Check sheet for the modelled part. Datum: model origin and axes. Units: mm. Face numbers are marked on the shaded views. A direction names the side the tool comes from. Give positions to 0.01 mm unless a question says otherwise; leave off trailing zeros. Order: outer loops, then holes, each group sorted by start corner. A loop starts at its lowest first (then second) coordinate and runs counter-clockwise, first axis right, second up.
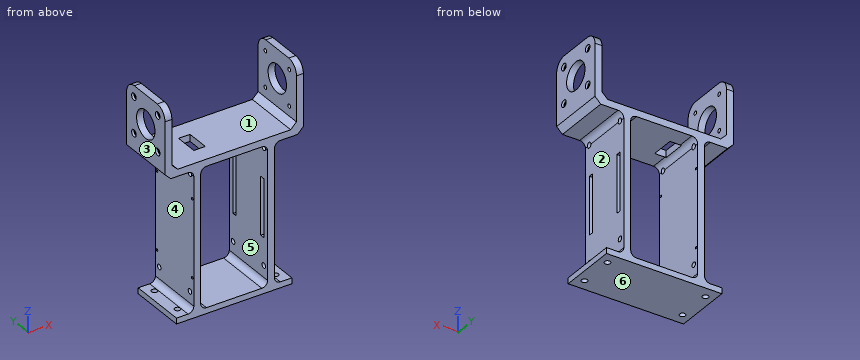
```python
from build123d import *

# Parameters (mm, degrees)
SKETCH1_W           = 120
SKETCH1_H           = 65
SKETCH1_W_2         = 108
SKETCH1_H_2         = 54
BOSS_EXTRUDE1_DEPTH = 50
SKETCH4_R           = 12
CUT_EXTRUDE1_DEPTH  = 156
SKETCH7_R           = 1.735318072
CUT_EXTRUDE2_DEPTH  = 156
SKETCH9_R           = 3
CUT_EXTRUDE3_DEPTH  = 2
CUT_EXTRUDE4_START  = -2
SKETCH10_R          = 3
CUT_EXTRUDE4_DEPTH  = 2
SKETCH11_W          = 6
SKETCH11_H          = 50
BOSS_EXTRUDE2_DEPTH = 120
SKETCH13_W          = 120
SKETCH13_H          = 5
CUT_EXTRUDE5_DEPTH  = 120
FILLET1_R           = 10
SKETCH14_W          = 100
SKETCH14_H          = 50
BOSS_EXTRUDE3_DEPTH = 5
SKETCH15_R          = 2.5
CUT_EXTRUDE6_DEPTH  = 18
SKETCH16_W          = 50
SKETCH16_H          = 4
CUT_EXTRUDE7_DEPTH  = 18
SKETCH17_R          = 1
CUT_EXTRUDE8_DEPTH  = 18
SKETCH18_W          = 10
SKETCH18_H          = 20
CUT_EXTRUDE9_DEPTH  = 18
SKETCH22_R          = 2.25
CUT_EXTRUDE13_DEPTH = 75
CHAMFER1_SIZE       = 5
CHAMFER2_SIZE       = 5
FILLET2_R           = 5


with BuildPart() as part:
    # Sketch1 → Boss-Extrude1 (new body)
    with BuildSketch(Plane(origin=(0, 0, 0), x_dir=(1, 0, 0), z_dir=(0, 1, 0))):
        with Locations((0, 2.5)):
            Rectangle(SKETCH1_W, SKETCH1_H)
        with Locations((0, 2)):
            Rectangle(SKETCH1_W_2, SKETCH1_H_2, mode=Mode.SUBTRACT)
    extrude(amount=BOSS_EXTRUDE1_DEPTH)

    # Sketch4 → Cut-Extrude1 (cut)
    with BuildSketch(Plane.ZY.offset(60)):
        with Locations((0, 25)):
            Circle(SKETCH4_R)
    extrude(amount=-CUT_EXTRUDE1_DEPTH, mode=Mode.SUBTRACT)

    # Sketch7 → Cut-Extrude2 (cut)
    with BuildSketch(Plane.ZY.offset(60)):
        with Locations((-15.5, 9.5)):
            Circle(SKETCH7_R)
        with Locations((-15.5, 40.5)):
            Circle(SKETCH7_R)
        with Locations((15.5, 9.5)):
            Circle(SKETCH7_R)
        with Locations((15.5, 40.5)):
            Circle(SKETCH7_R)
    extrude(amount=-CUT_EXTRUDE2_DEPTH, mode=Mode.SUBTRACT)

    # Sketch9 → Cut-Extrude3 (cut)
    with BuildSketch(Plane(origin=(60, 0, 0), x_dir=(0, 0, -1), z_dir=(1, 0, 0))):
        with Locations((15.5, 40.5)):
            Circle(SKETCH9_R)
        with Locations((15.5, 9.5)):
            Circle(SKETCH9_R)
        with Locations((-15.5, 9.5)):
            Circle(SKETCH9_R)
        with Locations((-15.5, 40.5)):
            Circle(SKETCH9_R)
    extrude(amount=-CUT_EXTRUDE3_DEPTH, mode=Mode.SUBTRACT)

    # Sketch10 → Cut-Extrude4 (cut)
    with BuildSketch(Plane.ZY.offset(60).offset(CUT_EXTRUDE4_START)):
        with Locations(Location((-15.5, 9.5, 0), (0, 0, 180))):
            Circle(SKETCH10_R)
        with Locations(Location((-15.5, 40.5, 0), (0, 0, 180))):
            Circle(SKETCH10_R)
        with Locations(Location((15.5, 40.5, 0), (0, 0, 180))):
            Circle(SKETCH10_R)
        with Locations(Location((15.5, 9.5, 0), (0, 0, 180))):
            Circle(SKETCH10_R)
    extrude(amount=CUT_EXTRUDE4_DEPTH, mode=Mode.SUBTRACT)

    # Sketch11 → Boss-Extrude2 (add)
    with BuildSketch(Plane(origin=(0, 0, -35), x_dir=(-1, 0, 0), z_dir=(0, 0, -1))):
        with Locations((-32, 25)):
            Rectangle(SKETCH11_W, SKETCH11_H)
        with Locations((32, 25)):
            Rectangle(SKETCH11_W, SKETCH11_H)
    extrude(amount=BOSS_EXTRUDE2_DEPTH)

    # Sketch13 → Cut-Extrude5 (cut)
    with BuildSketch(Plane(origin=(0, 50, 0), x_dir=(1, 0, 0), z_dir=(0, 1, 0))):
        with Locations((0, -27.5)):
            Rectangle(SKETCH13_W, SKETCH13_H)
    extrude(amount=-CUT_EXTRUDE5_DEPTH, mode=Mode.SUBTRACT)

    # Fillet1
    fillet1_edges = [part.edges().sort_by_distance(p)[0] for p in [
        (57, 0, 25),
        (-57, 0, 25),
        (57, 50, 25),
        (-57, 50, 25),
    ]]
    fillet(fillet1_edges, radius=FILLET1_R)

    # Sketch14 → Boss-Extrude3 (add)
    with BuildSketch(Plane(origin=(0, 0, -155), x_dir=(-1, 0, 0), z_dir=(0, 0, -1))):
        with Locations((0, 25)):
            Rectangle(SKETCH14_W, SKETCH14_H)
    extrude(amount=BOSS_EXTRUDE3_DEPTH)

    # Sketch15 → Cut-Extrude6 (cut)
    with BuildSketch(Plane(origin=(0, 0, -160), x_dir=(-1, 0, 0), z_dir=(0, 0, -1))):
        with Locations((-42.5, 10)):
            Circle(SKETCH15_R)
        with Locations((42.5, 10)):
            Circle(SKETCH15_R)
        with Locations((42.5, 40)):
            Circle(SKETCH15_R)
        with Locations((-42.5, 40)):
            Circle(SKETCH15_R)
    extrude(amount=-CUT_EXTRUDE6_DEPTH, mode=Mode.SUBTRACT)

    # Sketch16 → Cut-Extrude7 (cut)
    with BuildSketch(Plane(origin=(35, 0, 0), x_dir=(0, 0, -1), z_dir=(1, 0, 0))):
        with Locations((91.261804775, 43)):
            Rectangle(SKETCH16_W, SKETCH16_H)
        with Locations((91.261804775, 7)):
            Rectangle(SKETCH16_W, SKETCH16_H)
    extrude(amount=-CUT_EXTRUDE7_DEPTH, mode=Mode.SUBTRACT)

    # Sketch17 → Cut-Extrude8 (cut)
    with BuildSketch(Plane.ZY.offset(35)):
        with Locations(Location((-127, 2, 0), (0, 0, 270))):
            Circle(SKETCH17_R)
        with Locations(Location((-127, 48, 0), (0, 0, 270))):
            Circle(SKETCH17_R)
        with Locations(Location((-60, 2, 0), (0, 0, 270))):
            Circle(SKETCH17_R)
        with Locations(Location((-60, 48, 0), (0, 0, 270))):
            Circle(SKETCH17_R)
    extrude(amount=-CUT_EXTRUDE8_DEPTH, mode=Mode.SUBTRACT)

    # Sketch18 → Cut-Extrude9 (cut)
    with BuildSketch(Plane(origin=(0, 0, -35), x_dir=(-1, 0, 0), z_dir=(0, 0, -1))):
        with Locations((20, 25)):
            Rectangle(SKETCH18_W, SKETCH18_H)
    extrude(amount=-CUT_EXTRUDE9_DEPTH, mode=Mode.SUBTRACT)

    # Sketch22 → Cut-Extrude13 (cut)
    with BuildSketch(Plane.ZY.offset(35)):
        with Locations(Location((-140, 5, 0), (0, 0, 270))):
            Circle(SKETCH22_R)
        with Locations(Location((-140, 45, 0), (0, 0, 270))):
            Circle(SKETCH22_R)
        with Locations(Location((-40, 5, 0), (0, 0, 270))):
            Circle(SKETCH22_R)
        with Locations(Location((-40, 45, 0), (0, 0, 270))):
            Circle(SKETCH22_R)
    extrude(amount=-CUT_EXTRUDE13_DEPTH, mode=Mode.SUBTRACT)

    # Chamfer1
    chamfer1_edges = [part.edges().sort_by_distance(p)[0] for p in [
        (-60, 25, -35),
        (60, 25, -35),
    ]]
    chamfer(chamfer1_edges, length=CHAMFER1_SIZE)

    # Chamfer2
    chamfer2_edges = [part.edges().sort_by_distance(p)[0] for p in [
        (-54, 25, -29),
        (54, 25, -29),
    ]]
    chamfer(chamfer2_edges, length=CHAMFER2_SIZE)

    # Fillet2
    # the kernel refuses this fillet: 5 mm, written as the material it adds along each edge
    with BuildSketch(Plane(origin=(-29, 50, -155), x_dir=(1, 0, 0), z_dir=(0, -1, 0)), Plane(origin=(29, 0, -155), x_dir=(-1, 0, 0), z_dir=(0, 1, 0))) as fillet2_piece_1:
        with BuildLine():
            CenterArc((FILLET2_R, FILLET2_R), FILLET2_R, 180, 90)
            Line((0, FILLET2_R), (0, 0))
            Line((0, 0), (FILLET2_R, 0))
        make_face()
    extrude(amount=50)
    with BuildSketch(Plane(origin=(35, 50, -35), x_dir=(1, 0, 0), z_dir=(0, -1, 0))) as fillet2_piece_2_section:
        with BuildLine():
            CenterArc((FILLET2_R, -FILLET2_R), FILLET2_R, 90, 90)
            Line((0, -FILLET2_R), (0, 0))
            Line((0, 0), (FILLET2_R, 0))
        make_face()
    fillet2_piece_2 = extrude(amount=50, mode=Mode.PRIVATE)
    fillet2_piece_2 = fillet2_piece_2 - Plane(origin=(36.144503009, 45, -40), x_dir=(0, -1, 0), z_dir=(-1, 0, 0)) * Cylinder(2.25, 121, mode=Mode.PRIVATE)
    fillet2_piece_2 = fillet2_piece_2 - Plane(origin=(36.144503009, 5, -40), x_dir=(0, -1, 0), z_dir=(-1, 0, 0)) * Cylinder(2.25, 121, mode=Mode.PRIVATE)
    add(fillet2_piece_2)
    with BuildSketch(Plane(origin=(-29, 50, -35), x_dir=(0, 0, -1), z_dir=(0, -1, 0))) as fillet2_piece_3_section:
        with BuildLine():
            CenterArc((FILLET2_R, FILLET2_R), FILLET2_R, 180, 90)
            Line((0, FILLET2_R), (0, 0))
            Line((0, 0), (FILLET2_R, 0))
        make_face()
    fillet2_piece_3 = extrude(amount=50, mode=Mode.PRIVATE)
    fillet2_piece_3 = fillet2_piece_3 - Plane(origin=(-27.918643219, 45, -40), x_dir=(0, -1, 0), z_dir=(-1, 0, 0)) * Cylinder(2.25, 121, mode=Mode.PRIVATE)
    fillet2_piece_3 = split(fillet2_piece_3, bisect_by=Plane(origin=(-27.918643219, 35, -36.105806531), z_dir=(0, 1, 0)), keep=Keep.TOP, mode=Mode.PRIVATE)
    fillet2_piece_3 = split(fillet2_piece_3, bisect_by=Plane(origin=(-25, 42.450189762, -36.105806531), z_dir=(-1, 0, 0)), keep=Keep.TOP, mode=Mode.PRIVATE)
    add(fillet2_piece_3)
    with BuildSketch(Plane(origin=(-29, 50, -35), x_dir=(0, 0, -1), z_dir=(0, -1, 0))) as fillet2_piece_4_section:
        with BuildLine():
            CenterArc((FILLET2_R, FILLET2_R), FILLET2_R, 180, 90)
            Line((0, FILLET2_R), (0, 0))
            Line((0, 0), (FILLET2_R, 0))
        make_face()
    fillet2_piece_4 = extrude(amount=50, mode=Mode.PRIVATE)
    fillet2_piece_4 = split(fillet2_piece_4, bisect_by=Plane(origin=(-24.562912463, 35, -34.970154695), z_dir=(0, 1, 0)), keep=Keep.TOP, mode=Mode.PRIVATE)
    fillet2_piece_4 = split(fillet2_piece_4, bisect_by=Plane(origin=(-25, 42.5, -34.970154695), z_dir=(1, 0, 0)), keep=Keep.TOP, mode=Mode.PRIVATE)
    add(fillet2_piece_4)
    with BuildSketch(Plane(origin=(-29, 50, -35), x_dir=(0, 0, -1), z_dir=(0, -1, 0))) as fillet2_piece_5_section:
        with BuildLine():
            CenterArc((FILLET2_R, FILLET2_R), FILLET2_R, 180, 90)
            Line((0, FILLET2_R), (0, 0))
            Line((0, 0), (FILLET2_R, 0))
        make_face()
    fillet2_piece_5 = extrude(amount=50, mode=Mode.PRIVATE)
    fillet2_piece_5 = split(fillet2_piece_5, bisect_by=Plane(origin=(-27.938736848, 35, -36.15683257), z_dir=(0, -1, 0)), keep=Keep.TOP, mode=Mode.PRIVATE)
    fillet2_piece_5 = split(fillet2_piece_5, bisect_by=Plane(origin=(-27.938736848, 15, -36.15683257), z_dir=(0, 1, 0)), keep=Keep.TOP, mode=Mode.PRIVATE)
    fillet2_piece_5 = split(fillet2_piece_5, bisect_by=Plane(origin=(-25, 25, -36.15683257), z_dir=(-1, 0, 0)), keep=Keep.TOP, mode=Mode.PRIVATE)
    add(fillet2_piece_5)
    with BuildSketch(Plane(origin=(-29, 50, -35), x_dir=(0, 0, -1), z_dir=(0, -1, 0))) as fillet2_piece_6_section:
        with BuildLine():
            CenterArc((FILLET2_R, FILLET2_R), FILLET2_R, 180, 90)
            Line((0, FILLET2_R), (0, 0))
            Line((0, 0), (FILLET2_R, 0))
        make_face()
    fillet2_piece_6 = extrude(amount=50, mode=Mode.PRIVATE)
    fillet2_piece_6 = fillet2_piece_6 - Plane(origin=(-27.918643238, 5, -40), x_dir=(0, -1, 0), z_dir=(-1, 0, 0)) * Cylinder(2.25, 121, mode=Mode.PRIVATE)
    fillet2_piece_6 = split(fillet2_piece_6, bisect_by=Plane(origin=(-27.918643238, 15, -36.105806633), z_dir=(0, -1, 0)), keep=Keep.TOP, mode=Mode.PRIVATE)
    fillet2_piece_6 = split(fillet2_piece_6, bisect_by=Plane(origin=(-25, 7.54981005, -36.105806633), z_dir=(-1, 0, 0)), keep=Keep.TOP, mode=Mode.PRIVATE)
    add(fillet2_piece_6)
    with BuildSketch(Plane(origin=(-29, 50, -35), x_dir=(0, 0, -1), z_dir=(0, -1, 0))) as fillet2_piece_7_section:
        with BuildLine():
            CenterArc((FILLET2_R, FILLET2_R), FILLET2_R, 180, 90)
            Line((0, FILLET2_R), (0, 0))
            Line((0, 0), (FILLET2_R, 0))
        make_face()
    fillet2_piece_7 = extrude(amount=50, mode=Mode.PRIVATE)
    fillet2_piece_7 = split(fillet2_piece_7, bisect_by=Plane(origin=(-24.562912463, 15, -34.970154695), z_dir=(0, -1, 0)), keep=Keep.TOP, mode=Mode.PRIVATE)
    fillet2_piece_7 = split(fillet2_piece_7, bisect_by=Plane(origin=(-25, 7.5, -34.970154695), z_dir=(1, 0, 0)), keep=Keep.TOP, mode=Mode.PRIVATE)
    add(fillet2_piece_7)
    with BuildSketch(Plane(origin=(-35, 0, -35), x_dir=(-1, 0, 0), z_dir=(0, 1, 0))) as fillet2_piece_8_section:
        with BuildLine():
            CenterArc((FILLET2_R, -FILLET2_R), FILLET2_R, 90, 90)
            Line((0, -FILLET2_R), (0, 0))
            Line((0, 0), (FILLET2_R, 0))
        make_face()
    fillet2_piece_8 = extrude(amount=50, mode=Mode.PRIVATE)
    fillet2_piece_8 = fillet2_piece_8 - Plane(origin=(-36.144503009, 5, -40), x_dir=(0, -1, 0), z_dir=(-1, 0, 0)) * Cylinder(2.25, 121, mode=Mode.PRIVATE)
    fillet2_piece_8 = fillet2_piece_8 - Plane(origin=(-36.144503009, 45, -40), x_dir=(0, -1, 0), z_dir=(-1, 0, 0)) * Cylinder(2.25, 121, mode=Mode.PRIVATE)
    add(fillet2_piece_8)
    with BuildSketch(Plane(origin=(29, 0, -35), x_dir=(-1, 0, 0), z_dir=(0, 1, 0))) as fillet2_piece_9_section:
        with BuildLine():
            CenterArc((FILLET2_R, -FILLET2_R), FILLET2_R, 90, 90)
            Line((0, -FILLET2_R), (0, 0))
            Line((0, 0), (FILLET2_R, 0))
        make_face()
    fillet2_piece_9 = extrude(amount=50, mode=Mode.PRIVATE)
    fillet2_piece_9 = fillet2_piece_9 - Plane(origin=(27.855496991, 5, -40), x_dir=(0, -1, 0), z_dir=(-1, 0, 0)) * Cylinder(2.25, 121, mode=Mode.PRIVATE)
    fillet2_piece_9 = fillet2_piece_9 - Plane(origin=(27.855496991, 45, -40), x_dir=(0, -1, 0), z_dir=(-1, 0, 0)) * Cylinder(2.25, 121, mode=Mode.PRIVATE)
    add(fillet2_piece_9)
    with BuildSketch(Plane(origin=(-35, 0, -155), x_dir=(0, 0, 1), z_dir=(0, 1, 0)), Plane(origin=(35, 50, -155), x_dir=(0, 0, 1), z_dir=(0, -1, 0))) as fillet2_piece_10:
        with BuildLine():
            CenterArc((FILLET2_R, -FILLET2_R), FILLET2_R, 90, 90)
            Line((0, -FILLET2_R), (0, 0))
            Line((0, 0), (FILLET2_R, 0))
        make_face()
    extrude(amount=50)


solid = part.part
```
Q1. Tool access check on the marked faces 4, 5 and 6. Record the directions out of +Z, -Z, +X, -X, +Y, -Y that give a thin tool (end or side, any length) a straight path to the whole face; none if there is none.
Q2. Sectioned sample at B-B, the plane x = 42.5. Record the cut outline in (y, z).
Q3. Sectioned sample at A-A, the plane z = -134. Record the cut outline in (x, y), plus the area to 3 significant figures.
Q4. Draft check along Z on the marked faces 1, 2 and 3. Enter one of: pulls with the +Z half, pulls with the -Z half, needs draft (parallel to the pull), parting line crosses it, or undercut.
Q5. Sectioned sample at C-C, the plane z = 0. Record the cut outline in (x, y).
Q6. Material ranges on line 1 (Y direction, x = 58.8, z = 15.5); line 2 (Y direction, x = -55.6, z = -15.5); line 3 (X direction, y = 13, z = -97.5), recorded low to high.
Q7. Go/stop test with flat-tipped pins: P1, Ø2, axis at y = 40.5, z = 15.5, coming from the -X side; P2, Ø15, axis at y = 33.5, z = -72, coming from the -X side; P3, Ø4, axis at y = 23, z = -157, coming from the -X side; P4, Ø4, axis at y = 21, z = -75, coming from the +X side. Record where each tip stops, or that it passes through.
Q8. Sectioned sample at D-D, the plane y = 30. Count the separate pieces of the cut face and the enclosed holes in it, plus the area to 3 significant figures.
Filled in:
1. face 4: -X, +Y, -Y
1. face 5: +Y, -Y
1. face 6: -Z, +X, -X, +Y, -Y
2. outline: (0, -160) - (7.5, -160) - (7.5, -155) - (0, -155) - close; (0, -35) - (50, -35) - (50, -29) - (0, -29) - close; (12.5, -160) - (37.5, -160) - (37.5, -155) - (12.5, -155) - close; (42.5, -160) - (50, -160) - (50, -155) - (42.5, -155) - close
3. outline: (-35, 0) - (-29, 0) - (-29, 50) - (-35, 50) - close; (29, 0) - (35, 0) - (35, 50) - (29, 50) - close
3. area: 600 mm2
4. face 1: pulls with the +Z half
4. face 2: undercut
4. face 3: needs draft
5. outline: (-60, 0) - (-54, 0) - (-54, 13) - (-60, 13) - close; (-60, 37) - (-54, 37) - (-54, 50) - (-60, 50) - close; (54, 0) - (60, 0) - (60, 13) - (54, 13) - close; (54, 37) - (60, 37) - (60, 50) - (54, 50) - close
6. line 1: y = 0.01 to 6.5, 12.5 to 37.5, 43.5 to 49.99
6. line 2: y = 0 to 7.76, 11.24 to 38.76, 42.24 to 50
6. line 3: x = -35 to -29, 29 to 35
7. P1: passes through
7. P2: stops at x = -35
7. P3: stops at x = -50
7. P4: stops at x = 35
8. separate pieces: 3
8. enclosed holes: 0
8. area: 3,030 mm2
